For this review, use the dimensioned drawing (mm, ordinates from the lowest corner) and the shaded views. A direction names the side the tool comes from. Coordinates: 2 decimals unless noted, no trailing zeros. Loops run counter-clockwise (first coordinate to the right, second up) from the corner with the lowest first, then second, coordinate; pieces in that order, holes last. Notation, with made-up numbers: (36, -23) - (88, -23) arc R7 ccw to (88, -10) - close; hole circle Ø7 at (13, 20). An arc over 180 degrees is marked (long way). Answer in a Markdown table with one row per item. Add a question column.
(1) We need section B-B on y = 45.5. Write out the cut boundary in (x, z).
(2) We need section A-A on z = 1.7. Write out the cut boundary in (x, y), plus the area to 3 significant figures.
(3) Machinability: for the marked faces 4 and 5, which of the approach directions +Z, -Z, +X, -X, +Y, -Y give a long, thin tool a straight path to every point of the face, cutting with its end or side? Answer none if there is none.
(4) Mouldability with a two-part tool opening along X and no side actions: class the marked faces 1, 2 and 3 as +X half, -X half, draft (parallel to the pull), parting line (faces both ways), or undercut.
(5) For P1, Ø1.5, axis at y = 27, z = 1.5, coming from the -X side; P2, Ø9, axis at x = 39, y = 44, coming from the +Z side, all flat-tipped, find the tip position at first contact; note any pin that passes through.
(6) For line 1 along Y through (x, z) = (14.5, 0.35); line 2 along X through (y, z) = (22, 2.35); line 3 along Y through (x, z) = (32.5, 1.25), list the stretches that pass through material, from the lowest coordinate up.
(7) We need section C-C on x = 16. Write out the cut boundary in (y, z).
(8) We need section D-D on y = 6.5. Write out the cut boundary in (x, z).
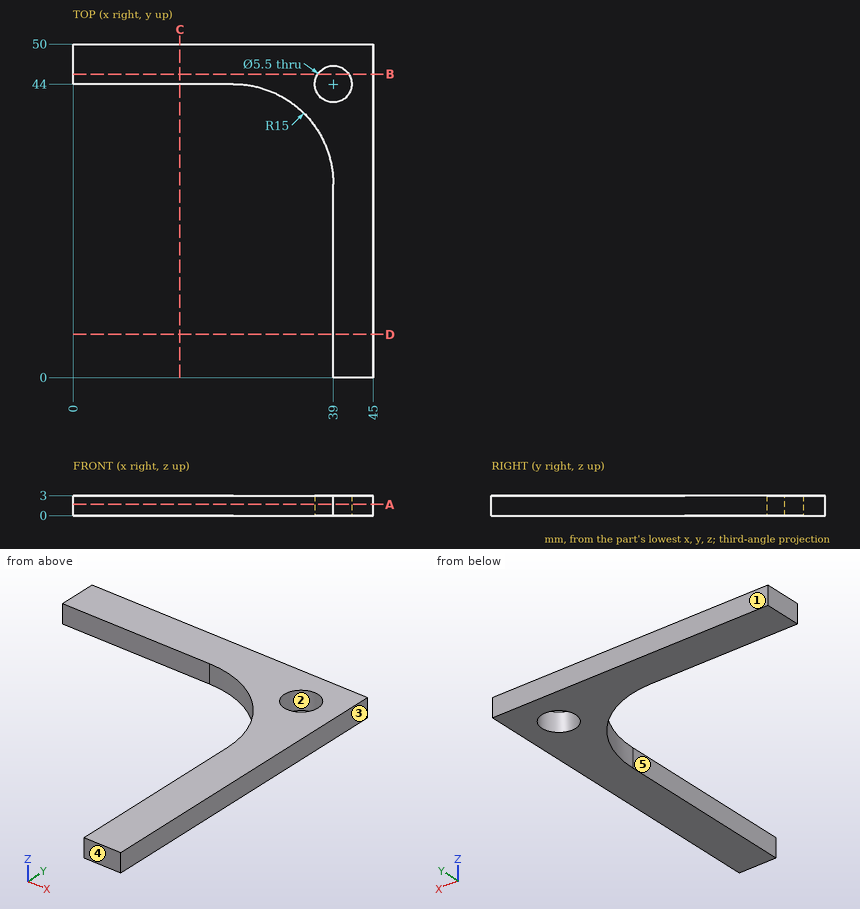
Outcome:
| question | item | result |
|---|---|---|
| 1 | outline | (0, 0) - (36.7, 0) - (36.7, 3) - (0, 3) - close; (41.3, 0) - (45, 0) - (45, 3) - (41.3, 3) - close |
| 2 | outline | (0, 44) - (24, 44) arc R15 cw to (39, 29) - (39, 0) - (45, 0) - (45, 50) - (0, 50) - close; hole circle Ø5.5 at (39, 44) |
| 2 | area | 559 mm² |
| 3 | face 4 | +Z, -Z, +X, -X, -Y |
| 3 | face 5 | +Z, -Z, -X, -Y |
| 4 | face 1 | draft |
| 4 | face 2 | undercut |
| 4 | face 3 | +X half |
| 5 | P1 | x = 39 |
| 5 | P2 | z = 3 |
| 6 | line 1 | 44 to 50 |
| 6 | line 2 | 39 to 45 |
| 6 | line 3 | 41.36 to 50 |
| 7 | outline | (44, 0) - (50, 0) - (50, 3) - (44, 3) - close |
| 8 | outline | (39, 0) - (45, 0) - (45, 3) - (39, 3) - close |
